from build123d import *

# Parameters (mm, degrees)
F1_DEPTH       = 63.5
F1_DEPTH_BACK  = 63.5
F4_DEPTH       = 3
F6_D           = 5.5
F6_CSINK_D     = 11.2
F6_CSINK_ANGLE = 90
F8_DEPTH       = 20
F9_DEPTH       = 20


with BuildPart() as f1:
    # F0 (on Front) → F1 (new body, two sides)
    with BuildSketch(Plane.XZ) as f1_sk:
        Polygon((-25.4, 5), (-25.4, 0), (25.4, 0), (25.4, 5), (16.498962309, 5), (20, 10), (-20, 10), (-16.498962309, 5), align=None)
    extrude(amount=F1_DEPTH)
    extrude(f1_sk.sketch, amount=-F1_DEPTH_BACK)

    # F3 (on face) → F4 (cut)
    with BuildSketch(Plane(origin=(0, 0, 0), x_dir=(1, 0, 0), z_dir=(0, 0, -1))):
        with BuildLine():
            Line((2, 22.5), (-2, 22.5))
            ThreePointArc((-2, 22.5), (-4.1213203436, 21.6213203436), (-5, 19.5))
            Line((-5, 19.5), (-5, -19.5))
            ThreePointArc((-5, -19.5), (-4.1213203436, -21.6213203436), (-2, -22.5))
            Line((-2, -22.5), (2, -22.5))
            ThreePointArc((2, -22.5), (4.1213203436, -21.6213203436), (5, -19.5))
            Line((5, -19.5), (5, 19.5))
            ThreePointArc((5, 19.5), (4.1213203436, 21.6213203436), (2, 22.5))
        make_face()
    extrude(amount=-F4_DEPTH, mode=Mode.SUBTRACT)

    # F6 (through all)
    with Locations(Plane.XY.offset(10)):
        with Locations((-10.5, 57.5), (10.5, 57.5), (-9.928368032, 29.5), (9.928368032, 29.5), (-9.928368032, -29.5), (9.928368032, -29.5), (-10.5, -57.5), (10.5, -57.5)):
            CounterSinkHole(F6_D / 2, F6_CSINK_D / 2, counter_sink_angle=F6_CSINK_ANGLE)

    # F7 (on face) → F8 (join)
    with BuildSketch(Plane.XZ.offset(63.5)):
        Polygon((35.4, 5), (25.4, 5), (0, 5), (0, 0), (10.570820421, 0), (30.4, -25), (35.4, -25), align=None)
        Polygon((0, 0), (0, 5), (-25.4, 5), (-35.4, 5), (-35.4, -25), (-30.4, -25), (-10.570820421, 0), align=None)
    extrude(amount=F8_DEPTH)

    # F9 (add): a face of the model
    f9_faces = [f1.faces().sort_by_distance(p)[0] for p in [
        (0, -63.5, 7.5799346399),
    ]]
    extrude(f9_faces, amount=F9_DEPTH)


solid = f1.part
Build history of the part. All positions in model axes, mm. A direction names the side the tool comes from. Round coordinates to 2 decimals unless told otherwise and drop trailing zeros. Write each loop counter-clockwise with the first axis right and the second up, starting at its lowest first coordinate (ties: lowest second). Pieces come first, ordered by that corner, then holes. Notation, with made-up numbers: (8.25, 10.5) - (20.25, 10.5) arc R17 ccw to (20.25, 20.5) - close; hole circle Ø9 at (52.5, 83.25). An arc over 180 degrees is marked (long way). Use CSV: the item, a comma, the result in double quotes.
(1) Band-saw the part on C-C (y = -3). Write the cut outline in (x, z).
Response:
outline,"(-25.4, 0) - (-5, 0) - (-5, 3) - (5, 3) - (5, 0) - (25.4, 0) - (25.4, 5) - (16.5, 5) - (20, 10) - (-20, 10) - (-16.5, 5) - (-25.4, 5) - close"
(2) Band-saw the part on B-B (z = -11). Write the cut outline in (x, y).
Response:
outline,"(-35.4, -83.5) - (-19.3, -83.5) - (-19.3, -63.5) - (-35.4, -63.5) - close; (19.3, -83.5) - (35.4, -83.5) - (35.4, -63.5) - (19.3, -63.5) - close"
(3) Wall check: line 1 (X direction, y = 29.5, z = 3.75); line 2 (X direction, y = 57.5, z = 4); line 3 (Y direction, x = 10.5, z = 3). Give the ranges that are in metal, low to high.
Response:
line 1,"-25.4 to -12.68, -7.18 to 7.18, 12.68 to 25.4"
line 2,"-25.4 to -13.25, -7.75 to 7.75, 13.25 to 25.4"
line 3,"-83.5 to -60.25, -54.75 to -32.19, -26.81 to 26.81, 32.19 to 54.75, 60.25 to 63.5"
(4) Band-saw the part on A-A (y = 29.5). Write the cut outline in (x, z), plus the area to 3 significant figures.
Response:
outline,"(-25.4, 0) - (-12.68, 0) - (-12.68, 7.15) - (-15.53, 10) - (-20, 10) - (-16.5, 5) - (-25.4, 5) - close; (-7.18, 0) - (7.18, 0) - (7.18, 7.15) - (4.33, 10) - (-4.33, 10) - (-7.18, 7.15) - close; (12.68, 0) - (25.4, 0) - (25.4, 5) - (16.5, 5) - (20, 10) - (15.53, 10) - (12.68, 7.15) - close"
area,"310 mm²"
(5) 3-axis set-ups, long thin cutter, end or side, ignore diameter. For faces 4 (the flat face through (0, -9, 10)), 5 (the flat face through (5, 0, 1)): which of +Z, -Z, +X, -X, +Y, -Y reach the whole face in a straight line?
Response:
face 4,"+Z, +X, -X, +Y, -Y"
face 5,"-Z"
(6) Band-saw the part on D-D (z = -21). Write the cut outline in (x, y), plus the area to 3 significant figures.
Response:
outline,"(-35.4, -83.5) - (-27.23, -83.5) - (-27.23, -63.5) - (-35.4, -63.5) - close; (27.23, -83.5) - (35.4, -83.5) - (35.4, -63.5) - (27.23, -63.5) - close"
area,"327 mm²"
(7) Mould opens along Y. For faces 1 (the cylindrical face through (4.14, -21.6, 1.48)), 2 (the flat face through (0, -83.5, 1)), 3 (the flat face through (33, -73, -25)) say: pulls with the +Y half, pulls with the -Y half, needs draft (parallel to the pull), parting line crosses it, or undercut.
Response:
face 1,"undercut"
face 2,"pulls with the -Y half"
face 3,"needs draft"
(8) Pin check, flat tips, straight feed: P1, Ø2, axis at y = -50, z = 2, coming from the +X side; P2, Ø10, axis at y = -53, z = -5.5, coming from the +X side; P3, Ø5, axis at x = 0.5, y = 2, coming from the -Z side; P4, Ø9, axis at x = 9.93, y = 29.5, coming from the +Z side. Stop position of each tip, or through.
Response:
P1,"x = 25.4"
P2,"through"
P3,"z = 3"
P4,"z = 8.9"
